Model file for the job. Use its own axes, mm. A direction names the side the tool comes from. Round coordinates to 2 decimals unless told otherwise and drop trailing zeros. Order: outer loops, then holes, each group sorted by start corner. A loop starts at its lowest first (then second) coordinate and runs counter-clockwise, first axis right, second up. Notation, with made-up numbers: (79, 62) - (86, 62) arc R20 cw to (86, 101) - close; hole circle Ø3 at (-24, 39). An arc over 180 degrees is marked (long way). Write item = value, one per line. Start each with the question number.
from build123d import *

# Parameters (mm, degrees)
DOME1_FACE_RADIUS  = 3.302
DOME1_HEIGHT       = 2.54
CUT_EXTRUDE4_DEPTH = 21.698272826
SEEDCUT_COUNT      = 8


# Read off the part's stored shape, not the designer's step: Cut-Revolve-Thin7
with BuildPart() as part:
    # Sketch1 → Revolve5 (revolve)
    with BuildSketch(Plane(origin=(0, 0, 0), x_dir=(0, 0, -1), z_dir=(1, 0, 0)), mode=Mode.PRIVATE) as revolve5_sk:
        Polygon((-7.325846616, 0), (-7.325846616, 7.493), (-4.785846616, 7.493), (-4.785846616, 5.08), (7.914153384, 5.08), (7.914153384, 0), align=None)
    revolve(revolve5_sk.sketch.rotate(Axis((0, 0, 20.020603184), (0, 0, -1)), 90), axis=Axis((0, 0, 20.020603184), (0, 0, -1)))

    # Sketch2 → Revolve12 (revolve)
    with BuildSketch(Plane(origin=(0, 0, 0), x_dir=(0, 0, -1), z_dir=(1, 0, 0))):
        with BuildLine():
            Line((-7.325846616, 0), (-21.775464383, 0))
            add(Edge.make_bspline(
                [(-7.325846616, 6.761687124), (-12.74249131, 6.612472482), (-17.889702324, 3.558506137), (-21.775464383, 0)],
                knots=[0, 0, 0, 0, 1, 1, 1, 1], degree=3))
            Line((-7.325846616, 6.761687124), (-7.325846616, 0))
        make_face()
    revolve(axis=Axis((0, 0, 22.807457961), (0, 0, -1)))

    # Cut-Revolve-Thin7 outline → Cut-Revolve-Thin7 (revolve, cut)
    with BuildSketch(Plane.XZ):
        Polygon((3.302, -6.136153384), (3.302, -7.914153384), (5.08, -7.914153384), (5.08, -1.564153384), align=None)
    revolve(axis=Axis((0, 0, 0), (0, 0, 1)), mode=Mode.SUBTRACT)

    # Dome1: a dome of height H over a round flat face of radius A is a cap of a sphere of radius (A * A + H * H) / (2 * H)
    dome1_r = (DOME1_FACE_RADIUS * DOME1_FACE_RADIUS + DOME1_HEIGHT * DOME1_HEIGHT) / (2 * DOME1_HEIGHT)
    dome1_base = Plane((0, 0, -7.914153384), z_dir=(0, 0, -1))
    with Locations(dome1_base.offset(DOME1_HEIGHT - dome1_r)):
        dome1_ball = Sphere(dome1_r, mode=Mode.PRIVATE)
    add(split(dome1_ball, bisect_by=dome1_base, keep=Keep.TOP, mode=Mode.PRIVATE))

    # Sketch6 → Cut-Extrude4 (cut, through all)
    with BuildSketch(Plane.XY.offset(7.325846616)):
        with BuildLine():
            Line((0, 7.127343562), (0.357140372, 7.484483934))
            ThreePointArc((0.357140372, 7.484483934), (0, 7.493), (-0.357140372, 7.484483934))
            Line((-0.357140372, 7.484483934), (0, 7.127343562))
        make_face()
    cut_extrude4 = extrude(amount=-CUT_EXTRUDE4_DEPTH, mode=Mode.SUBTRACT)

    # SeedCut: Cut-Extrude4 ×8 about axis
    seedcut_axis = Axis((0, 0, 0), (0, 0, 1))
    for i in range(1, SEEDCUT_COUNT):
        add(cut_extrude4.rotate(seedcut_axis, i * 360 / SEEDCUT_COUNT), mode=Mode.SUBTRACT)


solid = part.part
Item 1: Drop flat-ended pins along their axis: pin 1 (4 mm diameter, centred on x = 1, y = -4.5, fed in from -Z); pin 2 (7.5 mm diameter, centred on x = 2.5, y = -3.5, fed in from +Z); pin 3 (3 mm diameter, centred on x = 1, y = 5.5, fed in from +Z); pin 4 (7.5 mm diameter, centred on x = -1.5, y = -2.5, fed in from -Z). Give the stop position or say it passes through.
Item 2: Saw through at B-B, the plane z = -7.5. Give the cut face in (x, y).
Item 3: Which spindle directions (+Z, -Z, +X, -X, +Y, -Y) get a long thin tool onto all of the face, cutting with end or side? Do faces 1 (the face through (7, 1, 7.326)), 2 (the face through (3.05, -1.26, -7.04)), 3 (the face through (-2.9, 6.91, 6.04)). Say none if no direction does.
Item 4: Saw through at A-A, the plane z = 6. Give the cut face in (x, y).
Item 5: Saw through at C-C, the plane z = 2.5. Give the cut face in (x, y), then the cut area to 3 significant figures.
Item 6: Probe L1, parallel to Z at x = -1.25, y = 7; L2, parallel to Z at x = -5, y = -2; L3, parallel to X at y = -4.25, z = -1. List the from-to ranges inside material, lowest first.
Check sheet entries:
q1.pin_1 = -9.24
q1.pin_2 = 21.16
q1.pin_3 = 16.19
q1.pin_4 = -10.45
q2.outline = circle Ø6.6 at (0, 0)
q3.face_1 = +Z
q3.face_2 = -Z
q3.face_3 = +Z, -Z, -X, +Y
q4.outline = (-7.48, -0.36) arc R7.49 ccw to (-5.54, -5.04) - (-5.04, -5.04) - (-5.04, -5.54) arc R7.49 ccw to (-0.36, -7.48) - (0, -7.13) - (0.36, -7.48) arc R7.49 ccw to (5.04, -5.54) - (5.04, -5.04) - (5.54, -5.04) arc R7.49 ccw to (7.48, -0.36) - (7.13, 0) - (7.48, 0.36) arc R7.49 ccw to (5.54, 5.04) - (5.04, 5.04) - (5.04, 5.54) arc R7.49 ccw to (0.36, 7.48) - (0, 7.13) - (-0.36, 7.48) arc R7.49 ccw to (-5.04, 5.54) - (-5.04, 5.04) - (-5.54, 5.04) arc R7.49 ccw to (-7.48, 0.36) - (-7.13, 0) - close
q5.outline = circle Ø10.16 at (0, 0)
q5.area = 81.1 mm2
q6.L1 = 4.79 to 7.33
q6.L2 = 4.79 to 13.53
q6.L3 = -2.78 to 2.78
